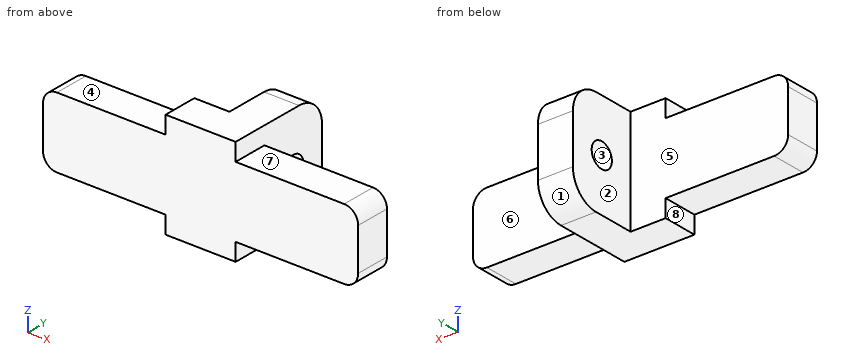
from build123d import *

# Parameters (mm, degrees)
SKETCH_3_W                  = 45
SKETCH_3_H                  = 10
EXTRUDE_2_DEPTH             = 5
SKETCH_4_W                  = 10
SKETCH_4_H                  = 15
EXTRUDE_3_DEPTH             = 10
EXTRUDE_3_DIRECTION_2_REACH = 25.585
SKETCH_5_R                  = 1.75
CUT_EXTRUDE_1_DEPTH         = 10
FILLET_2_R                  = 2
FILLET_1_R                  = 4
SKETCH_8_W                  = 20
SKETCH_8_H                  = 10
CUT_EXTRUDE_2_DEPTH         = 5


with BuildPart() as part:
    # 草图3 → 凸台-拉伸2 (new body)
    with BuildSketch(Plane(origin=(0, 0, 0), x_dir=(1, 0, 0), z_dir=(0, 1, 0))):
        Rectangle(SKETCH_3_W, SKETCH_3_H)
    extrude(amount=EXTRUDE_2_DEPTH)

    # 草图4 → 凸台-拉伸3 (add)
    with BuildSketch(Plane(origin=(0, 5, 0), x_dir=(1, 0, 0), z_dir=(0, 1, 0))):
        Rectangle(SKETCH_4_W, SKETCH_4_H)
    extrude(amount=EXTRUDE_3_DEPTH)

    # 凸台-拉伸3 direction 2: up to this face of the body (flat: up to its plane)
    extrude_3_direction_2_end = Plane(part.part.faces().sort_by_distance((0, 0, 0))[0])
    # 草图4 → 凸台-拉伸3 direction 2 (add, up to the picked face)
    with BuildSketch(Plane(origin=(0, 5, 0), x_dir=(1, 0, 0), z_dir=(0, 1, 0)), mode=Mode.PRIVATE) as extrude_3_direction_2_sk1:
        Rectangle(SKETCH_4_W, SKETCH_4_H)
    extrude_3_direction_2_tool1 = split(extrude(extrude_3_direction_2_sk1.sketch, amount=-EXTRUDE_3_DIRECTION_2_REACH, mode=Mode.PRIVATE), bisect_by=extrude_3_direction_2_end, keep=Keep.BOTH, mode=Mode.PRIVATE)
    add(extrude_3_direction_2_tool1.solids().sort_by(Axis((0, 5, 0), (0, -1, 0)))[0])

    # 草图5 → 切除-拉伸1 (cut)
    with BuildSketch(Plane.ZY.offset(5)):
        with Locations((0, 10)):
            Circle(SKETCH_5_R)
    extrude(amount=-CUT_EXTRUDE_1_DEPTH, mode=Mode.SUBTRACT)

    # 圆角2
    fillet_2_edges = [part.edges().sort_by_distance(p)[0] for p in [
        (22.5, 2.5, 5),
        (-22.5, 2.5, 5),
        (-22.5, 2.5, -5),
        (22.5, 2.5, -5),
    ]]
    fillet(fillet_2_edges, radius=FILLET_2_R)

    # 圆角1
    fillet_1_edges = [part.edges().sort_by_distance(p)[0] for p in [
        (0, 15, -7.5),
        (0, 15, 7.5),
    ]]
    fillet(fillet_1_edges, radius=FILLET_1_R)

    # 草图8 → 切除-拉伸2 (cut)
    with BuildSketch(Plane.ZY.offset(5)):
        with Locations((0, 10)):
            Rectangle(SKETCH_8_W, SKETCH_8_H)
    extrude(amount=-CUT_EXTRUDE_2_DEPTH, mode=Mode.SUBTRACT)


solid = part.part
Here's how the part is built. I have some questions about the finished solid (model axes, mm). Face numbers are marked on the shaded views. A direction names the side the tool comes from. Round coordinates to 2 decimals unless told otherwise and drop trailing zeros. Loops run counter-clockwise (first coordinate to the right, second up) from the corner with the lowest first, then second, coordinate; pieces in that order, holes last. Notation, with made-up numbers: (-20, 64.5) - (19, 64.5) arc R30 ccw to (19, 92.5) - close; hole circle Ø5 at (40, -39.75). An arc over 180 degrees is marked (long way). One line per question, with ' | ' between items. Start each with the question number.
Q1. Please list where these lines run through material, in increasing order: line 1 (Y direction, x = 3.45, z = 0); line 2 (X direction, y = 14.5, z = -0.75). Write a range as [from, to].
Q2. I want a section at B-B (z = -0.25). Write out the boundary of the cut face in (x, y), then the cut area to 3 significant figures.
Q3. Will these pins go through, and if not, where does the flat tip stop? pin 1 (4 mm diameter, centred on x = 7.5, z = 0, fed in from -Y); pin 2 (4.5 mm diameter, centred on y = 10, z = 0, fed in from -X); pin 3 (5.5 mm diameter, centred on x = 13, y = 3, fed in from +Z); pin 4 (3 mm diameter, centred on x = 12, z = 2, fed in from +Y).
Q4. For the marked faces 4, 5, 6, 7 and 8, which set-ups out of +Z, -Z, +X, -X, +Y, -Y let a thin tool reach every point of the face, with its end or its side?
Q5. I want a section at A-A (y = 10). Write out the boundary of the cut face in (x, z), then the cut area to 3 significant figures.
Q6. I want a section at C-C (y = 3). Write out the boundary of the cut face in (x, z), then the cut area to 3 significant figures.
Q7. We'd pull the mould along Z, two halves only. Please class the marked faces 1, 2 and 3: +Z half, -Z half, draft (parallel to the pull), parting line (faces both ways), or undercut.
Q8. I want a section at D-D (z = 2.5). Write out the boundary of the cut face in (x, y), then the cut area to 3 significant figures.
Response values:
1) line 1: y = [0, 8.25], [11.75, 15] | line 2: x = [0, 5]
2) outline: (-22.5, 0) - (22.5, 0) - (22.5, 5) - (5, 5) - (5, 8.27) - (0, 8.27) - (0, 5) - (-22.5, 5) - close; (0, 11.73) - (5, 11.73) - (5, 15) - (0, 15) - close | area: 258 mm²
3) pin 1: stops at y = 0 | pin 2: stops at x = 0 | pin 3: stops at z = 5 | pin 4: stops at y = 5
4) face 4: +Z, -X, +Y, -Y | face 5: +Z, -Z, -X, +Y | face 6: +Z, -Z, +X, +Y | face 7: +Z, +X, +Y, -Y | face 8: -Z, -X, +Y, -Y
5) outline: (0, -7.5) - (5, -7.5) - (5, -1.75) - (0, -1.75) - close; (0, 1.75) - (5, 1.75) - (5, 7.5) - (0, 7.5) - close | area: 57.5 mm²
6) outline: (-22.5, -3) arc R2 ccw to (-20.5, -5) - (-5, -5) - (-5, -7.5) - (5, -7.5) - (5, -5) - (20.5, -5) arc R2 ccw to (22.5, -3) - (22.5, 3) arc R2 ccw to (20.5, 5) - (5, 5) - (5, 7.5) - (-5, 7.5) - (-5, 5) - (-20.5, 5) arc R2 ccw to (-22.5, 3) - close | area: 497 mm²
7) face 1: -Z half | face 2: draft | face 3: undercut
8) outline: (-22.5, 0) - (22.5, 0) - (22.5, 5) - (5, 5) - (5, 15) - (0, 15) - (0, 5) - (-22.5, 5) - close | area: 275 mm²
